Autodesk Inventor part; units mm, degrees
ref_plane "YZ Plane" through (0, 0, 0) normal (1, 0, 0) x (0, 1, 0)
ref_plane "XZ Plane" through (0, 0, 0) normal (0, 1, 0) x (-1, 0, 0)
ref_plane "XY Plane" through (0, 0, 0) normal (0, 0, 1) x (1, 0, 0)
sketch "Эскиз1" plane through (0, 0, 0) normal (0, 1, 0) x (-1, 0, 0)
  line L0 (97.2595, 134.1284) -> (12.2595, 134.1284)
  line L1 (12.2595, 134.1284) -> (12.2595, -53.8716)
  line L2 (12.2595, -53.8716) -> (97.2595, -53.8716)
  line L3 (97.2595, -53.8716) -> (97.2595, 134.1284)
  line L4 (12.2595, 97.1284) -> (8.2595, 97.1284)
  line L5 (8.2595, 97.1284) -> (8.2595, 7.1284)
  line L6 (8.2595, 7.1284) -> (12.2595, 7.1284)
  line L7 (12.2595, 7.1284) -> (12.2595, 97.1284)
  line L8 (69.7595, 138.1284) -> (39.7595, 138.1284)
  line L9 (39.7595, 138.1284) -> (39.7595, 134.1284)
  line L10 (39.7595, 134.1284) -> (69.7595, 134.1284)
  line L11 (69.7595, 134.1284) -> (69.7595, 138.1284)
  line L12 (69.7595, -53.8716) -> (39.7595, -53.8716)
  line L13 (39.7595, -53.8716) -> (39.7595, -57.8716)
  line L14 (39.7595, -57.8716) -> (69.7595, -57.8716)
  line L15 (69.7595, -57.8716) -> (69.7595, -53.8716)
  line L16 (54.7595, -53.8716) -> (54.7595, -83.5129) construction
  point P0 (-14.3828, -135.2029)
  point P1 (-14.3828, -200.4773)
  point P2 (-14.3828, -47.8079)
  point P3 (-14.3828, 17.4664)
  point P4 (-10.7565, -263.2131)
  point P5 (-3.5038, -263.2131)
  point P6 (-3.5038, 232.8717)
  point P7 (-10.7565, 232.8717)
  point P8 (-3.5038, 79.8397)
  point P9 (-10.7565, 79.8397)
  point P10 (-14.3828, 17.4664)
  point P11 (-14.3828, -47.8079)
  point P12 (-10.7565, -110.1811)
  point P13 (-3.5038, -110.1811)
  point P14 (69.7595, 134.1284)
  point P15 (54.7595, -57.8716)
  point P16 (54.7595, 138.1284)
  dimension "d12" = 4
  dimension "d13" = 90
  dimension "d14" = 85
  dimension "d16" = 37
  dimension "d17" = 30
  dimension "d18" = 4
  dimension "d23" = 61
extrude "Выдавливание1" add sketch "Эскиз1" along normal blind 4
properties part number "стенка 3"
Verification items for the finished model (mm, model axes). A direction names the side the tool comes from. Coordinates: 2 decimals unless noted, no trailing zeros. Order: outer loops, then holes, each group sorted by start corner. A loop starts at its lowest first (then second) coordinate and runs counter-clockwise, first axis right, second up.
1. Sectioned sample at B-B, the plane z = 125.5. Record the cut outline in (x, y), and give its area (3 significant figures).
Results found:
outline: (-97.26, 0) - (-12.26, 0) - (-12.26, 4) - (-97.26, 4) - close
area: 340 mm2
2. Set-up check for faces 1 (the face through (-10, 2, 7.128)), 2 (the face through (-12.26, 2, 116)), 3 (the face through (-83, 2, -53.872)), 4 (the face through (-69.76, 2, 136)): record each of +Z, -Z, +X, -X, +Y, -Y from which the full face is reachable in a straight line by a thin tool's end or side.
Results found:
face 1: -Z, +X, +Y, -Y
face 2: +Z, +X, +Y, -Y
face 3: -Z, -X, +Y, -Y
face 4: +Z, -X, +Y, -Y
3. Go/stop test with flat-tipped pins: pin 1 Ø2 at (x, y) = (-86, 1.5) entering from -Z; pin 2 Ø2 at (x, y) = (-22.5, 1) entering from +Z; pin 3 Ø1.2 at (y, z) = (2.5, -55) entering from +X; pin 4 Ø5 at (x, z) = (-64.5, 37.5) entering from -Y. Record where each tip stops, or that it passes through.
Results found:
pin 1: stops at z = -53.87
pin 2: stops at z = 134.13
pin 3: stops at x = -39.76
pin 4: stops at y = 0
4. Scan lines: line 1 (Z direction, x = -78, y = 1.1); line 2 (X direction, y = 1.25, z = -17). Record each from-to range of solid material in increasing order.
Results found:
line 1: z = -53.87 to 134.13
line 2: x = -97.26 to -12.26
5. Sectioned sample at A-A, the plane y = 1.3. Record the cut outline in (x, z), and give its area (3 significant figures).
Results found:
outline: (-97.26, -53.87) - (-69.76, -53.87) - (-69.76, -57.87) - (-39.76, -57.87) - (-39.76, -53.87) - (-12.26, -53.87) - (-12.26, 7.13) - (-8.26, 7.13) - (-8.26, 97.13) - (-12.26, 97.13) - (-12.26, 134.13) - (-39.76, 134.13) - (-39.76, 138.13) - (-69.76, 138.13) - (-69.76, 134.13) - (-97.26, 134.13) - close
area: 16,600 mm2
6. Sectioned sample at C-C, the plane x = -85.5. Record the cut outline in (y, z).
Results found:
outline: (0, -53.87) - (4, -53.87) - (4, 134.13) - (0, 134.13) - close
